from build123d import *

# Parameters (mm, degrees)
F0_W     = 76.2
F0_H     = 76.2
F1_DEPTH = 76.2
F2_R     = 5.08
F3_T     = -2.54


# Not quite as in the source:
# - a shell that OpenCascade refuses in one call is made with other operations: the cavity is built on its own and cut out


with BuildPart() as f1:
    # F0 (on Top) → F1 (new body)
    with BuildSketch(Plane.XY):
        with Locations((7.7656768262, 2.775496821)):
            Rectangle(F0_W, F0_H)
    extrude(amount=F1_DEPTH)

    # F2
    f2_edges = [f1.edges().sort_by_distance(p)[0] for p in [
        (7.765677, -35.324503, 76.2),
        (45.865677, 2.775497, 76.2),
        (7.765677, 40.875497, 76.2),
        (-30.334323, 2.775497, 76.2),
        (45.865677, -35.324503, 38.1),
        (-30.334323, -35.324503, 38.1),
        (45.865677, 40.875497, 38.1),
        (-30.334323, 40.875497, 38.1),
    ]]
    fillet(f2_edges, radius=F2_R)

    # F3: a shell. OpenCascade refuses it in one call, so the cavity is built on its own and cut out:
    # the body offset inwards by the wall thickness, plus a prism from it out through each open face.
    f3_core = offset(f1.part, amount=F3_T, mode=Mode.PRIVATE)
    f3_exits = [f3_core.faces().sort_by_distance(p)[0] for p in [
        (7.765677, 2.775497, 73.66),
    ]]
    add(f3_core, mode=Mode.SUBTRACT)
    extrude(f3_exits, amount=-F3_T, mode=Mode.SUBTRACT)


solid = f1.part
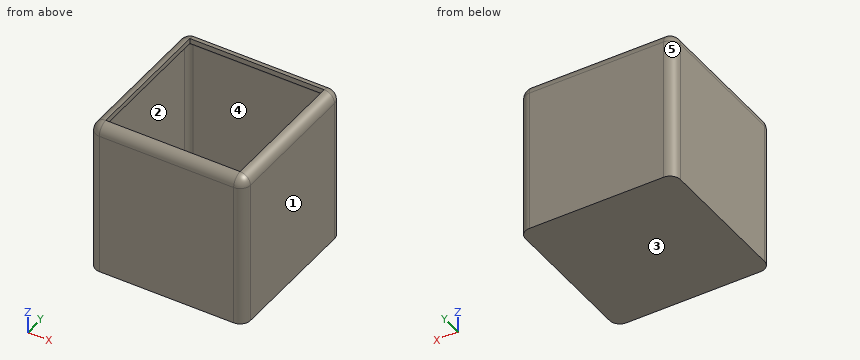
Read the model definition and answer for the solid it produces. Units are mm, in the model's axes. Face numbers are marked on the shaded views. A direction names the side the tool comes from. Round coordinates to 2 decimals unless told otherwise and drop trailing zeros. Write each loop counter-clockwise with the first axis right and the second up, starting at its lowest first coordinate (ties: lowest second). Pieces come first, ordered by that corner, then holes.
Q1. Find section C-C on y = 9. Determine the outline of the cut face in (x, z).
Values:
outline: (-30.33, 0) - (45.87, 0) - (45.87, 71.12) arc R5.08 ccw to (40.79, 76.2) - (40.79, 73.66) arc R2.54 cw to (43.33, 71.12) - (43.33, 2.54) - (-27.79, 2.54) - (-27.79, 71.12) arc R2.54 cw to (-25.25, 73.66) - (-25.25, 76.2) arc R5.08 ccw to (-30.33, 71.12) - close
Q2. The mould has two halves that part along Z. Classify the marked faces 1, 2 and 3: released by +Z, released by -Z, zero draft, split by the parting line, or undercut.
Values:
face 1: zero draft
face 2: undercut
face 3: released by -Z
Q3. Straight lines are drawn through the part: line 1 (Y direction, x = -4, z = 19.5); line 2 (X direction, y = -14, z = 27.5); line 3 (Z direction, x = 30, y = -20). For each, find the intervals that lie inside material, in ascending order.
Values:
line 1: y = -35.32 to -32.78, 38.34 to 40.88
line 2: x = -30.33 to -27.79, 43.33 to 45.87
line 3: z = 0 to 2.54
Q4. Flat-ended cylindrical pins translate along their axes: P1, Ø2, axis at x = 20.5, z = 74.5, coming from the +Y side; P2, Ø1.5, axis at x = 19.5, y = 17, coming from the -Z side; P3, Ø1.3, axis at y = -4, z = 75, coming from the -X side; P4, Ø21.5, axis at x = 0, y = -2.5, coming from the +Z side. Find the tip coordinate at first contact, or state that the pin passes through.
Values:
P1: stops at y = 40.28
P2: stops at z = 0
P3: stops at x = -29.18
P4: stops at z = 2.54
Q5. Find section A-A on z = 49.5. Determine the outline of the cut face in (x, y), and give its area (3 significant figures).
Values:
outline: (-30.33, -30.24) arc R5.08 ccw to (-25.25, -35.32) - (40.79, -35.32) arc R5.08 ccw to (45.87, -30.24) - (45.87, 35.8) arc R5.08 ccw to (40.79, 40.88) - (-25.25, 40.88) arc R5.08 ccw to (-30.33, 35.8) - close; hole (-27.79, -30.24) arc R2.54 ccw to (-25.25, -32.78) - (40.79, -32.78) arc R2.54 ccw to (43.33, -30.24) - (43.33, 35.8) arc R2.54 ccw to (40.79, 38.34) - (-25.25, 38.34) arc R2.54 ccw to (-27.79, 35.8) - close
area: 732 mm2
Q6. A tool of negligible diameter and unlimited length cuts with its end or side. For the marked faces 4 and 5, from which of +Z, -Z, +X, -X, +Y, -Y can it reach the whole face along a straight path? Write none if from no direction.
Values:
face 4: none
face 5: +Z, -Z, -X, +Y
Q7. Find section B-B on x = -17.5. Determine the outline of the cut face in (y, z), and give its area (3 significant figures).
Values:
outline: (-35.32, 0) - (40.88, 0) - (40.88, 71.12) arc R5.08 ccw to (35.8, 76.2) - (35.8, 73.66) arc R2.54 cw to (38.34, 71.12) - (38.34, 2.54) - (-32.78, 2.54) - (-32.78, 71.12) arc R2.54 cw to (-30.24, 73.66) - (-30.24, 76.2) arc R5.08 ccw to (-35.32, 71.12) - close
area: 572 mm2
